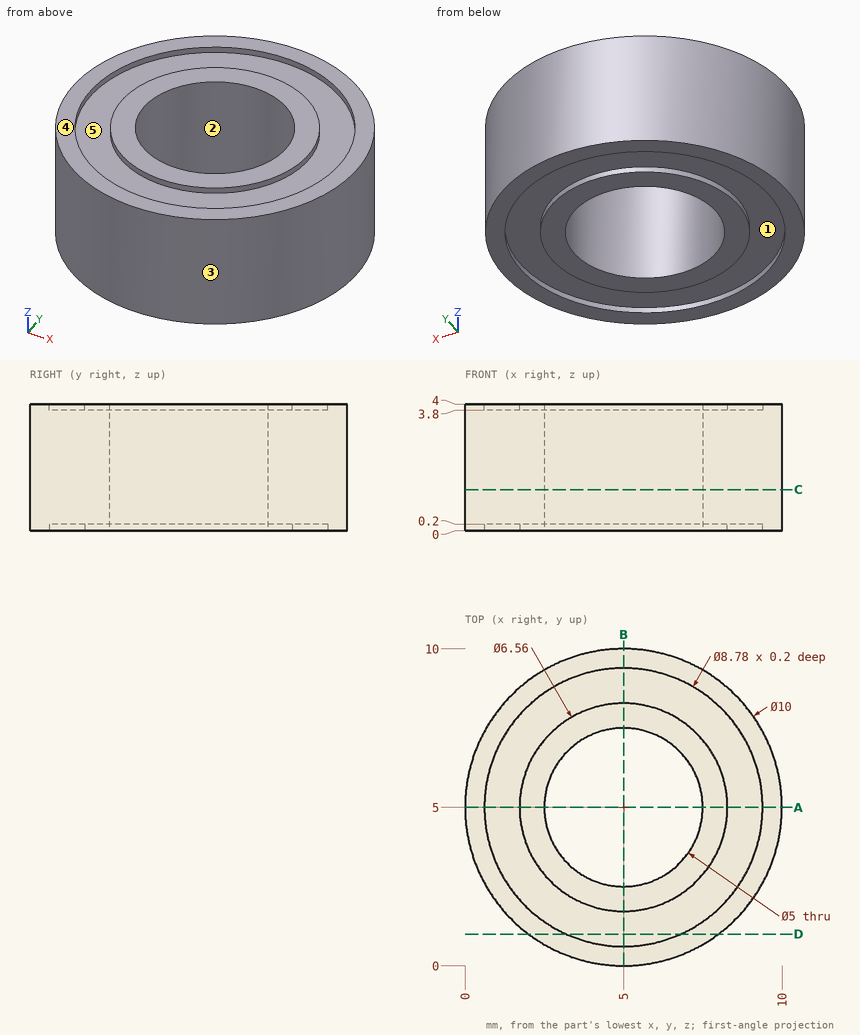
Job drawing, mm, ordinate dimensions from the low corner. One solid piece. A direction names the side the tool comes from. Give positions to 0.01 mm unless a question says otherwise; leave off trailing zeros. Loops run counter-clockwise (first coordinate to the right, second up) from the corner with the lowest first, then second, coordinate; pieces in that order, holes last.
Item 1: Which spindle directions (+Z, -Z, +X, -X, +Y, -Y) get a long thin tool onto all of the face, cutting with end or side? Do the marked faces 1 and 2. Say none if no direction does.
Answers follow:
face 1: -Z
face 2: +Z, -Z
Item 2: Slice it at A-A, the plane y = 5. List the corners of the cut face in (x, z).
Answers follow:
outline: (0, 0) - (0.61, 0) - (0.61, 0.2) - (1.72, 0.2) - (1.72, 0) - (2.5, 0) - (2.5, 4) - (1.72, 4) - (1.72, 3.8) - (0.61, 3.8) - (0.61, 4) - (0, 4) - close; (7.5, 0) - (8.28, 0) - (8.28, 0.2) - (9.39, 0.2) - (9.39, 0) - (10, 0) - (10, 4) - (9.39, 4) - (9.39, 3.8) - (8.28, 3.8) - (8.28, 4) - (7.5, 4) - close
Item 3: Pull direction Y, two halves, no side cores. Call the marked faces 3, 4 and 5: released by +Y, released by -Y, zero draft, split by the parting line, or undercut.
Answers follow:
face 3: split by the parting line
face 4: zero draft
face 5: undercut
Item 4: Flat gauge pins, fed straight in: pin 1 (2 mm diameter, centred on y = 4.5, z = 2, fed in from +X); pin 2 (1.5 mm diameter, centred on x = 9, z = 1, fed in from -Y); pin 3 (4.5 mm diameter, centred on x = 5, y = 5, fed in from -Z); pin 4 (1.5 mm diameter, centred on x = 8, z = 2, fed in from +Y). Where does each tip first touch, or does it go through?
Answers follow:
pin 1: stops at x = 10
pin 2: stops at y = 1.2
pin 3: passes through
pin 4: stops at y = 9.47
Item 5: Drill centre lines: line 1 (Y direction, x = 5, z = 0.15); line 2 (Y direction, x = 5, z = 1.2); line 3 (Z direction, x = 2.25, y = 7). Where is each one in solid material? Low to high.
Answers follow:
line 1: y = 0 to 0.61, 1.72 to 2.5, 7.5 to 8.28, 9.39 to 10
line 2: y = 0 to 2.5, 7.5 to 10
line 3: z = 0.2 to 3.8
Item 6: Slice it at C-C, the plane z = 1.3. List the corners of the cut face in (x, y).
Answers follow:
outline: circle Ø10 at (5, 5); hole circle Ø5 at (5, 5)
Item 7: Slice it at D-D, the plane y = 1. List the corners of the cut face in (x, z), and give its area (3 significant figures).
Answers follow:
outline: (2, 0) - (3.19, 0) - (3.19, 0.2) - (6.81, 0.2) - (6.81, 0) - (8, 0) - (8, 4) - (6.81, 4) - (6.81, 3.8) - (3.19, 3.8) - (3.19, 4) - (2, 4) - close
area: 22.6 mm2
